from build123d import *

# Parameters (mm, degrees)
SKETCH1_R           = 23.2
SKETCH1_R_2         = 12.2
BOSS_EXTRUDE1_DEPTH = 10
SKETCH2_R           = 12.2
BOSS_EXTRUDE2_DEPTH = 3
SKETCH3_R           = 7.5
CUT_EXTRUDE1_DEPTH  = 3
SKETCH4_R           = 23.2
SKETCH4_R_2         = 20
BOSS_EXTRUDE3_DEPTH = 6
CUT_EXTRUDE3_DEPTH  = 59
SKETCH8_R           = 23.8
SKETCH8_R_2         = 23.2
BOSS_EXTRUDE4_DEPTH = 16


with BuildPart() as part:
    # Sketch1 → Boss-Extrude1 (new body)
    with BuildSketch(Plane(origin=(0, 0, 0), x_dir=(1, 0, 0), z_dir=(0, 1, 0))):
        Circle(SKETCH1_R)
        Circle(SKETCH1_R_2, mode=Mode.SUBTRACT)
    extrude(amount=BOSS_EXTRUDE1_DEPTH)

    # Sketch2 → Boss-Extrude2 (add)
    with BuildSketch(Plane.XZ):
        Circle(SKETCH2_R)
    extrude(amount=-BOSS_EXTRUDE2_DEPTH)

    # Sketch3 → Cut-Extrude1 (cut)
    with BuildSketch(Plane(origin=(0, 3, 0), x_dir=(1, 0, 0), z_dir=(0, 1, 0))):
        Circle(SKETCH3_R)
    extrude(amount=-CUT_EXTRUDE1_DEPTH, mode=Mode.SUBTRACT)

    # Sketch4 → Boss-Extrude3 (add)
    with BuildSketch(Plane(origin=(0, 10, 0), x_dir=(1, 0, 0), z_dir=(0, 1, 0))):
        Circle(SKETCH4_R)
        Circle(SKETCH4_R_2, mode=Mode.SUBTRACT)
    extrude(amount=BOSS_EXTRUDE3_DEPTH)

    # Sketch6 → Cut-Extrude3 (cut)
    with BuildSketch(Plane(origin=(0, 10, 0), x_dir=(1, 0, 0), z_dir=(0, 1, 0))):
        with BuildLine():
            Line((15.848028, 12.2), (9.066422, 12.2))
            ThreePointArc((9.066422, 12.2), (15.2, 0), (9.066422, -12.2))
            Line((9.066422, -12.2), (15.848028, -12.2))
            ThreePointArc((15.848028, -12.2), (20, 0), (15.848028, 12.2))
        make_face()
        with BuildLine():
            ThreePointArc((-9.066422, -12.2), (-15.2, 0), (-9.066422, 12.2))
            Line((-9.066422, 12.2), (-15.848028, 12.2))
            ThreePointArc((-15.848028, 12.2), (-20, 0), (-15.848028, -12.2))
            Line((-15.848028, -12.2), (-9.066422, -12.2))
        make_face()
    extrude(amount=-CUT_EXTRUDE3_DEPTH, mode=Mode.SUBTRACT)

    # Sketch8 → Boss-Extrude4 (add)
    with BuildSketch(Plane(origin=(0, 16, 0), x_dir=(1, 0, 0), z_dir=(0, 1, 0))):
        Circle(SKETCH8_R)
        Circle(SKETCH8_R_2, mode=Mode.SUBTRACT)
    extrude(amount=-BOSS_EXTRUDE4_DEPTH)


solid = part.part
Can you work these out from the model? Positions are in its coordinate system, mm. A direction names the side the tool comes from. Coordinates: 2 decimals unless noted, no trailing zeros. Write each loop counter-clockwise with the first axis right and the second up, starting at its lowest first coordinate (ties: lowest second). Pieces come first, ordered by that corner, then holes. Notation, with made-up numbers: (-27.75, 53) - (10.25, 53) arc R25 cw to (10.25, 71) - close; hole circle Ø5 at (86.25, 43). An arc over 180 degrees is marked (long way). Return JSON: item names as keys, results as strings. Group by question number.
Item 1: I'm going to push flat-ended pins straight in: pin 1 Ø6 at (x, y) = (-18.5, 5) entering from -Z; pin 2 Ø1 at (y, z) = (8.5, -4) entering from -X; pin 3 Ø6 at (y, z) = (10, 14.5) entering from -X. Where does each tip first touch, or does it pass through?
Item 2: Please list where these lines run through material, in increasing order: probe 1 along X at (y, z) = (13.7, 0); probe 2 along Z at (x, y) = (0, 6.5).
Item 3: Which directions (+Z, -Z, +X, -X, +Y, -Y) give clear straight access to the entire face, cutting with the end or side of a thin tool? Please do faces 1 (the face through (5, 3, 6)), 2 (the face through (-12, 5, -12.2)), 3 (the face through (-6, 0, -6)).
Item 4: If we section it at C-C (z = 0): Write out the boundary of the cut face in (x, y), then the cut area to 3 significant figures.
Item 5: If we section it at B-B (y = 6): Write out the boundary of the cut face in (x, z), then the cut area to 3 significant figures.
Item 6: If we section it at A-A (x = 0): Write out the boundary of the cut face in (y, z).
Item 7: If we section it at D-D (z = -10): Write out the boundary of the cut face in (x, y).
Item 8: We'd pull the mould along X, two halves only. Please class faces 4 (the face through (-13, 5, 12.2)), 5 (the face through (-5, 16, -20)), 6 (the face through (-17.542, 8.112, -16.085)): pulls with the +X half, pulls with the -X half, needs draft (parallel to the pull), parting line crosses it, or undercut.
Return value:
{
 "1": {"pin 1": "stops at z = -18.06", "pin 2": "stops at x = -23.54", "pin 3": "stops at x = -20.84"},
 "2": {"probe 1": "x = -23.8 to -20, 20 to 23.8", "probe 2": "z = -23.8 to -12.2, 12.2 to 23.8"},
 "3": {"face 1": "+Y", "face 2": "+Y, -Y", "face 3": "+Z, -Z, +X, -X, -Y"},
 "4": {"outline": "(-23.8, 0) - (-20, 0) - (-20, 16) - (-23.8, 16) - close; (-15.2, 0) - (-7.5, 0) - (-7.5, 3) - (-12.2, 3) - (-12.2, 10) - (-15.2, 10) - close; (7.5, 0) - (15.2, 0) - (15.2, 10) - (12.2, 10) - (12.2, 3) - (7.5, 3) - close; (20, 0) - (23.8, 0) - (23.8, 16) - (20, 16) - close", "area": "210 mm^2"},
 "5": {"outline": "circle Ø47.6 at (0, 0); hole (-15.85, -12.2) - (-9.07, -12.2) arc R15.2 cw to (-9.07, 12.2) - (-15.85, 12.2) arc R20 ccw to start; hole circle Ø24.4 at (0, 0); hole (9.07, -12.2) - (15.85, -12.2) arc R20 ccw to (15.85, 12.2) - (9.07, 12.2) arc R15.2 cw to start", "area": "1,050 mm^2"},
 "6": {"outline": "(0, -23.8) - (16, -23.8) - (16, -20) - (10, -20) - (10, -12.2) - (3, -12.2) - (3, -7.5) - (0, -7.5) - close; (0, 7.5) - (3, 7.5) - (3, 12.2) - (10, 12.2) - (10, 20) - (16, 20) - (16, 23.8) - (0, 23.8) - close"},
 "7": {"outline": "(-21.6, 0) - (-17.32, 0) - (-17.32, 16) - (-21.6, 16) - close; (-11.45, 0) - (11.45, 0) - (11.45, 10) - (6.99, 10) - (6.99, 3) - (-6.99, 3) - (-6.99, 10) - (-11.45, 10) - close; (17.32, 0) - (21.6, 0) - (21.6, 16) - (17.32, 16) - close"},
 "8": {"face 4": "undercut", "face 5": "needs draft", "face 6": "parting line crosses it"}
}
